The model under review builds one solid part; all positions refer to its coordinate system, in mm. Face numbers are marked on the shaded views. A direction names the side the tool comes from. Round coordinates to 2 decimals unless told otherwise and drop trailing zeros. Loops run counter-clockwise (first coordinate to the right, second up) from the corner with the lowest first, then second, coordinate; pieces in that order, holes last. Notation, with made-up numbers: (36.5, 55) -> (40.5, 55) arc R18 ccw to (40.5, 78) -> close; hole circle Ø11 at (52.25, -12.5). An arc over 180 degrees is marked (long way). Write each question's results on one line, items separated by ' | '. Start each with the question number.
Item 1: We need section B-B (y = 0.5). Give the boundary of the cut face in (x, z).
Item 2: We need section C-C (z = -2.5). Give the boundary of the cut face in (x, y).
Item 3: Clearance check with flat-ended pins moving along their axes: pin 1 Ø2 at (x, z) = (-6, -20) entering from +Y; pin 2 Ø0.8 at (y, z) = (1, -17) entering from -X; pin 3 Ø8 at (x, z) = (-20, -21) entering from -Y; pin 4 Ø1.2 at (x, y) = (0.5, 4.5) entering from -Z. State where each tip first meets the part, or that it passes through.
Item 4: We need section A-A (x = -3.5). Give the boundary of the cut face in (y, z).
Item 5: Mouldability with a two-part tool opening along X and no side actions: class the marked faces 1, 2, 3 and 4 as pulls with the +X half, pulls with the -X half, needs draft (parallel to the pull), parting line crosses it, or undercut.
Item 6: We need section D-D (y = 7.5). Give the boundary of the cut face in (x, z), and give its area (3 significant figures).
Item 7: Tool access review of the marked faces 5, 6 and 7: name each direction out of +Z, -Z, +X, -X, +Y, -Y from which nothing blocks a thin tool from reaching the whole face with its end or side.
Item 8: For L1, parallel to Z at x = -3.5, y = 1.2; L2, parallel to X at y = 1.05, z = -21.5; L3, parallel to X at y = 7, z = -13, list the stretches that pass through material, from the lowest coordinate up. Write a range as from..to.
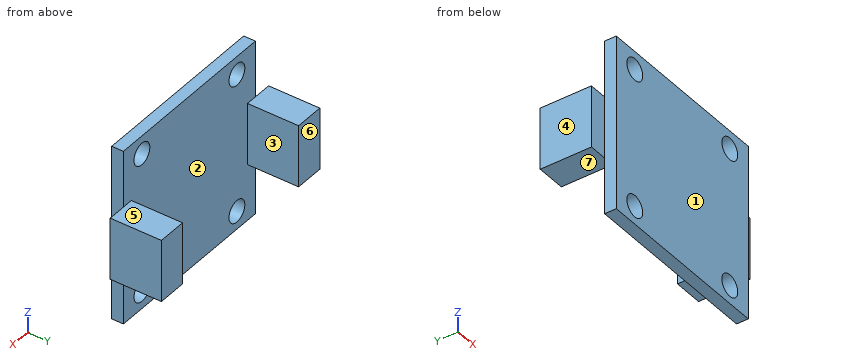
Autodesk Inventor part; units mm, degrees
ref_plane "YZ Plane" through (0, 0, 0) normal (1, 0, 0) x (0, 1, 0)
ref_plane "XZ Plane" through (0, 0, 0) normal (0, 1, 0) x (-1, 0, 0)
ref_plane "XY Plane" through (0, 0, 0) normal (0, 0, 1) x (1, 0, 0)
sketch "Sketch1" plane through (0, 0, 0) normal (0, 1, 0) x (-1, 0, 0)
  line L0 (0, 0) -> (25, 0)
  line L1 (25, 0) -> (25, -24)
  line L2 (25, -24) -> (0, -24)
  line L3 (0, -24) -> (0, 0)
  dimension "d0" = 24
  dimension "d1" = 25
extrude "Extrusion1" add sketch "Sketch1" along normal blind 1.6
sketch "Sketch2" plane through (0, 1.6, 0) normal (0, 1, 0) x (1, 0, 0)
  line L0 (-23.5, 7.75) -> (-27.5, 7.75)
  line L1 (-27.5, 7.75) -> (-27.5, 16.25)
  line L2 (-27.5, 16.25) -> (-23.5, 16.25)
  line L3 (-23.5, 16.25) -> (-23.5, 7.75)
  line L4 (-1.5, 7.75) -> (2.5, 7.75)
  line L5 (2.5, 7.75) -> (2.5, 16.25)
  line L6 (2.5, 16.25) -> (-1.5, 16.25)
  line L7 (-1.5, 16.25) -> (-1.5, 7.75)
  line L8 (-25, 0) -> (0, 0)
  line L9 (0, 24) -> (-25, 24)
  line L10 (0, 0) -> (0, 24)
  line L11 (-25, 24) -> (-25, 0)
  dimension "d4" = 8.5
  dimension "d5" = 7.75
  dimension "d6" = 7.75
  dimension "d8" = 4
  dimension "d9" = 8.5
  dimension "d10" = 7.75
  dimension "d11" = 2.5
  dimension "d13" = 4
  dimension "d14" = 2.5
extrude "Extrusion2" add sketch "Sketch2" along normal blind 7 contours L0 L11 L2 L3 | L0 L1 L2 L11 | L10 L6 L5 L4 | L4 L7 L6 L10
sketch "Sketch3" plane through (0, 1.6, 0) normal (0, 1, 0) x (1, 0, 0)
  line L0 (-25, 7.75) -> (-25, 0)
  line L1 (-25, 0) -> (0, 0)
  point P0 (-21.5, 2.5)
  point P1 (-21.5, 21.5)
  point P2 (-3.5, 2.5)
  point P3 (-3.5, 21.5)
  dimension "d17" = 3.5
  dimension "d18" = 2.5
  dimension "d21" = 19
  dimension "d24" = 18
hole "Hole1" at (-21.5, 1.6, -2.5) at (-21.5, 1.6, -21.5) at (-3.5, 1.6, -2.5) at (-3.5, 1.6, -21.5) direction (0, -1, 0) diameter 3 end through all
properties part number "Mock Board"
Here are the results:
1) outline: (-25, -24) -> (0, -24) -> (0, 0) -> (-25, 0) -> close; hole circle Ø3 at (-21.5, -21.5); hole circle Ø3 at (-21.5, -2.5); hole circle Ø3 at (-3.5, -21.5); hole circle Ø3 at (-3.5, -2.5)
2) outline: (-25, 0) -> (-23, 0) -> (-23, 1.6) -> (-25, 1.6) -> close; (-20, 0) -> (-5, 0) -> (-5, 1.6) -> (-20, 1.6) -> close; (-2, 0) -> (0, 0) -> (0, 1.6) -> (-2, 1.6) -> close
3) pin 1: stops at y = 1.6 | pin 2: stops at x = -25 | pin 3: stops at y = 0 | pin 4: stops at z = -16.25
4) outline: (0, -24) -> (1.6, -24) -> (1.6, -23) -> (0, -23) -> close; (0, -20) -> (1.6, -20) -> (1.6, -4) -> (0, -4) -> close; (0, -1) -> (1.6, -1) -> (1.6, 0) -> (0, 0) -> close
5) face 1: needs draft | face 2: undercut | face 3: undercut | face 4: pulls with the -X half
6) outline: (-27.5, -16.25) -> (-23.5, -16.25) -> (-23.5, -7.75) -> (-27.5, -7.75) -> close; (-1.5, -16.25) -> (2.5, -16.25) -> (2.5, -7.75) -> (-1.5, -7.75) -> close | area: 68.0 mm2
7) face 5: +Z, +X, -X, +Y | face 6: +Z, -Z, +X, -X, +Y | face 7: -Z, +X, -X, +Y
8) L1: z = -24..-23, -20..-4, -1..0 | L2: x = -25..-23, -20..-5, -2..0 | L3: x = -27.5..-23.5, -1.5..2.5
